from build123d import *

# Parameters (mm, degrees)
SKETCH_1_R      = 5
EXTRUDE_1_DEPTH = 14
SKETCH_4_R      = 0.5
EXTRUDE_2_DEPTH = 2
FILLET_2_R      = 1


with BuildPart() as part:
    # 草图1 → 凸台-拉伸1 (new body)
    with BuildSketch(Plane.XY):
        Circle(SKETCH_1_R)
    extrude(amount=EXTRUDE_1_DEPTH)

    # 草图3 → 切除-旋转1 (revolve, cut)
    with BuildSketch(Plane(origin=(0, 0, 0), x_dir=(1, 0, 0), z_dir=(0, 1, 0))):
        Polygon((-5.273110547, -2.186263047), (-3.629051397, -3.830322197), (-3.629051397, -9.985928365), (-5.273110547, -11.629987515), align=None)
    revolve(axis=Axis((0, 0, -0.7), (0, 0, 1)), mode=Mode.SUBTRACT)

    # 草图4 → 凸台-拉伸2 (add)
    with BuildSketch(Plane.XY):
        with Locations((-2.54, 0)):
            Circle(SKETCH_4_R)
        with Locations(Location((2.54, 0, 0), (0, 0, 180))):
            Circle(SKETCH_4_R)
    extrude(amount=-EXTRUDE_2_DEPTH)

    # 圆角2
    fillet_2_edges = [part.edges().sort_by_distance(p)[0] for p in [
        (-5, 0, 0),
        (-5, 0, 14),
        (0, -5, 2.459373595),
        (0, -5, 11.356876968),
    ]]
    fillet(fillet_2_edges, radius=FILLET_2_R)


solid = part.part
Design review of the part built by this model. Coordinates are the model's own, in mm. A direction names the side the tool comes from. Round coordinates to 2 decimals unless told otherwise and drop trailing zeros. Write each loop counter-clockwise with the first axis right and the second up, starting at its lowest first coordinate (ties: lowest second). Pieces come first, ordered by that corner, then holes. Notation, with made-up numbers: (24.25, 3.25) - (60.25, 3.25) arc R27 cw to (60.25, 27.25) - close; hole circle Ø3 at (80, 25). An arc over 180 degrees is marked (long way). Use a Markdown table: item, result. Add a question column.
1. We need section A-A (z = -0.5). State the section outline as (x, y) points.
2. Mouldability with a two-part tool opening along Z and no side actions: class faces 3 (the face through (0.79, 3.54, 6.95)), 4 (the face through (3.04, -0.02, -0.99)), 5 (the face through (-2.5, 0, -2)) as +Z half, -Z half, draft (parallel to the pull), parting line (faces both ways), or undercut.
3. For faces 1 (the face through (-3.04, 0.02, -0.99)), 2 (the face through (4.77, 1.5, 1.52)), list the 3-axis set-ups (+Z, -Z, +X, -X, +Y, -Y) from which the entire face can be reached by the end or side of a thin tool; tool diameter is ignored.
4. We need section B-B (z = 6.5). State the section outline as (x, y) points, then the cut area to 3 significant figures.
5. We need section C-C (z = 1.75). State the section outline as (x, y) points, then the cut area to 3 significant figures.
6. Wall thickness on probe 1 along Z at (x, y) = (-1, 2.5); probe 2 along Z at (x, y) = (4.25, -1.5); probe 3 along Z at (x, y) = (3.5, -3.5): over which ranges is each line inside the solid? List them lowest first.
7. Clearance check with flat-ended pins moving along their axes: pin 1 (4 mm diameter, centred on x = 1.5, z = 9.5, fed in from +Y); pin 2 (1 mm diameter, centred on x = -1.5, z = 3, fed in from +Y); pin 3 (3 mm diameter, centred on x = -3.5, z = 10.5, fed in from -Y). State where each tip first meets the part, or that it passes through.
Output:
| question | item | result |
|---|---|---|
| 1 | outline | circle Ø1 at (-2.54, 0); circle Ø1 at (2.54, 0) |
| 2 | face 3 | undercut |
| 2 | face 4 | draft |
| 2 | face 5 | -Z half |
| 3 | face 1 | -Z |
| 3 | face 2 | +Z, -Z |
| 4 | outline | circle Ø7.26 at (0, 0) |
| 4 | area | 41.4 mm2 |
| 5 | outline | circle Ø10 at (0, 0) |
| 5 | area | 78.5 mm2 |
| 6 | probe 1 | z = 0 to 14 |
| 6 | probe 2 | z = 0.14 to 2.95, 10.86 to 13.86 |
| 6 | probe 3 | z = 0.69 to 2.36, 11.46 to 13.31 |
| 7 | pin 1 | stops at y = 4.85 |
| 7 | pin 2 | stops at y = 4.69 |
| 7 | pin 3 | stops at y = -4.36 |
